from build123d import *

# Parameters (mm, degrees)
F1_DEPTH = 25.4
F3_DEPTH = 203.2
F4_W     = 177.8
F4_H     = 88.9
F5_DEPTH = 101.6
F7_DEPTH = 22.225
F8_W     = 136.525
F8_H     = 190.5
F9_DEPTH = 22.225


with BuildPart() as f1:
    # F0 (on Top) → F1 (new body)
    with BuildSketch(Plane.XY):
        Polygon((30.969309, -60.027699), (30.969309, -136.227699), (208.769309, -136.227699), (208.769309, 117.772301), (-146.830691, 117.772301), (-146.830691, -60.027699), align=None)
    extrude(amount=F1_DEPTH)

    # F2 (on face) → F3 (join)
    with BuildSketch(Plane.XY.offset(25.4)):
        Polygon((-146.830691, 117.772301), (-146.830691, 3.472301), (-121.430691, 3.472301), (-121.430691, 92.372301), (-7.130691, 92.372301), (-7.130691, 117.772301), (-121.430691, 117.772301), align=None)
    extrude(amount=F3_DEPTH)

    # F4 (on face) → F5 (join)
    with BuildSketch(Plane.XY.offset(25.4)):
        with Locations((-57.930691, -15.577699)):
            Rectangle(F4_W, F4_H)
    extrude(amount=F5_DEPTH)

    # F6 (on face) → F7 (cut)
    with BuildSketch(Plane.YZ.offset(-121.430691)):
        Polygon((92.372301, 215.9), (3.472301, 215.9), (3.472301, 127), (28.872301, 127), (28.872301, 25.4), (92.372301, 25.4), (92.372301, 127), align=None)
    extrude(amount=-F7_DEPTH, mode=Mode.SUBTRACT)

    # F8 (on face) → F9 (cut)
    with BuildSketch(Plane.XZ.offset(-92.372301)):
        with Locations((-75.393191, 120.65)):
            Rectangle(F8_W, F8_H)
    extrude(amount=-F9_DEPTH, mode=Mode.SUBTRACT)


solid = f1.part
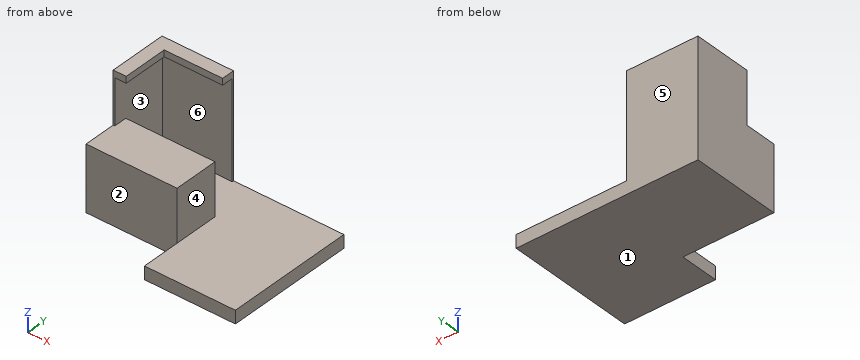
Model file for the job. Use its own axes, mm. Face numbers are marked on the shaded views. A direction names the side the tool comes from. Give positions to 0.01 mm unless a question says otherwise; leave off trailing zeros. Loops run counter-clockwise (first coordinate to the right, second up) from the corner with the lowest first, then second, coordinate; pieces in that order, holes last. Notation, with made-up numbers: (-2, -4) -> (12, -4) arc R16 cw to (12, 21) -> close; hole circle Ø10 at (22.5, 27). An arc over 180 degrees is marked (long way). Use a Markdown table: item, result. Add a question column.
(1) Slice it at D-D on y = 56.5. List the corners of the cut face in (x, z).
(2) Wall check: line 1 along Y through (x, z) = (-19.5, 85); line 2 along X through (y, z) = (-116, 21); line 3 along Z through (x, y) = (-111, 20.5). Give the ranges that are in metal, low to high.
(3) Mould opens along Y. For the marked faces 1, 2 and 3 say: +Y half, -Y half, draft (parallel to the pull), parting line (faces both ways), or undercut.
(4) Slice it at C-C on x = -69. List the corners of the cut face in (y, z), and give its area (3 significant figures).
(5) Slice it at B-B on z = 18. List the corners of the cut face in (x, y).
(6) Drop flat-ended pins along their axis: pin 1 Ø12.5 at (y, z) = (111, 164.5) entering from +X; pin 2 Ø7.5 at (x, z) = (-134, 172.5) entering from -Y; pin 3 Ø4 at (x, y) = (-92.5, -6.5) entering from +Z. Give the stop position or say it passes through.
(7) Tool access for the marked faces 4, 5 and 6: list every direction of +Z, -Z, +X, -X, +Y, -Y with a clear straight run to the whole face (end or side of a thin tool).
(8) Slice it at A-A on y = 10. List the corners of the cut face in (x, z).
Filled sheet:
| question | item | result |
|---|---|---|
| 1 | outline | (-146.83, 0) -> (208.77, 0) -> (208.77, 25.4) -> (-143.66, 25.4) -> (-143.66, 215.9) -> (-121.43, 215.9) -> (-121.43, 228.6) -> (-146.83, 228.6) -> close |
| 2 | line 1 | -60.03 to 28.87, 114.6 to 117.77 |
| 2 | line 2 | 30.97 to 208.77 |
| 2 | line 3 | 0 to 127 |
| 3 | face 1 | draft |
| 3 | face 2 | -Y half |
| 3 | face 3 | undercut |
| 4 | outline | (-60.03, 0) -> (117.77, 0) -> (117.77, 228.6) -> (92.37, 228.6) -> (92.37, 215.9) -> (114.6, 215.9) -> (114.6, 25.4) -> (28.87, 25.4) -> (28.87, 127) -> (-60.03, 127) -> close |
| 4 | area | 14,500 mm2 |
| 5 | outline | (-146.83, -60.03) -> (30.97, -60.03) -> (30.97, -136.23) -> (208.77, -136.23) -> (208.77, 117.77) -> (-146.83, 117.77) -> close |
| 6 | pin 1 | x = -7.13 |
| 6 | pin 2 | y = 114.6 |
| 6 | pin 3 | z = 127 |
| 7 | face 4 | +Z, +X, +Y, -Y |
| 7 | face 5 | +Z, -Z, +X, -X, +Y |
| 7 | face 6 | +X |
| 8 | outline | (-146.83, 0) -> (208.77, 0) -> (208.77, 25.4) -> (30.97, 25.4) -> (30.97, 127) -> (-143.66, 127) -> (-143.66, 215.9) -> (-121.43, 215.9) -> (-121.43, 228.6) -> (-146.83, 228.6) -> close |
